Can you work these out from the model? Positions are in its coordinate system, mm. Round coordinates to 2 decimals unless told otherwise and drop trailing zeros. Loops run counter-clockwise (first coordinate to the right, second up) from the corner with the lowest first, then second, coordinate; pieces in that order, holes last. Notation, with made-up numbers: M 53,4.5 L 103,4.5 A19 ccw 103,31.5 Z; hole C -10,-33.5 d6. An arc over 180 degrees is marked long. Return JSON: item names as keys, results as strings.
```python
from build123d import *

# Parameters (mm, degrees)
BOSS_EXTRUDE1_DEPTH      = 1.5875
BOSS_EXTRUDE1_DEPTH_BACK = 1.5875
SKETCH1_W                = 6.35
SKETCH1_H                = 19.05
SKETCH1_R                = 1.5875
FILLET1_R                = 3.175


with BuildPart() as part:
    # Sketch1 → Boss-Extrude1 (new, two sides: drawn at the far end of the back side and taken through both)
    with BuildSketch(Plane(origin=(0, 0, 0), x_dir=(0, 0, -1), z_dir=(1, 0, 0)).offset(-BOSS_EXTRUDE1_DEPTH_BACK)):
        with Locations((0, -6.35)):
            Rectangle(SKETCH1_W, SKETCH1_H)
        Circle(SKETCH1_R, mode=Mode.SUBTRACT)
        with Locations((0, -12.7)):
            Circle(SKETCH1_R, mode=Mode.SUBTRACT)
    extrude(amount=BOSS_EXTRUDE1_DEPTH + BOSS_EXTRUDE1_DEPTH_BACK)

    # Fillet1
    fillet1_edges = [part.edges().sort_by_distance(p)[0] for p in [
        (0, -15.875, -3.175),
        (0, -15.875, 3.175),
        (0, 3.175, -3.175),
        (0, 3.175, 3.175),
    ]]
    fillet(fillet1_edges, radius=FILLET1_R - 0.0001)  # a hair under: the kernel refuses the full size


solid = part.part
```
Q1. Suppose I cut it at D-D, the plane z = 0.5. Please give me the cut outline in (x, y), plus the area to 3 significant figures.
Results:
{"outline": "M -1.59,-15.84 L 1.59,-15.84 L 1.59,-14.21 L -1.59,-14.21 Z; M -1.59,-11.19 L 1.59,-11.19 L 1.59,-1.51 L -1.59,-1.51 Z; M -1.59,1.51 L 1.59,1.51 L 1.59,3.14 L -1.59,3.14 Z", "area": "41.1 mm2"}
Q2. Suppose I cut it at B-B, the plane z = -1. Please give me the cut outline in (x, y).
Results:
{"outline": "M -1.59,-15.71 L 1.59,-15.71 L 1.59,-13.93 L -1.59,-13.93 Z; M -1.59,-11.47 L 1.59,-11.47 L 1.59,-1.23 L -1.59,-1.23 Z; M -1.59,1.23 L 1.59,1.23 L 1.59,3.01 L -1.59,3.01 Z"}
Q3. If I drill on line 1 along Y through (x, z) = (0.25, 0) (1 decimal); line 2 along Y through (x, z) = (0, 0.5); line 3 along Y through (x, z) = (-1.3, 2.75), over which ranges is the centre line in solid material (lowest first)?
Results:
{"line 1": "y = -15.9 to -14.3, -11.1 to -1.6, 1.6 to 3.2", "line 2": "y = -15.84 to -14.21, -11.19 to -1.51, 1.51 to 3.14", "line 3": "y = -14.29 to 1.59"}
Q4. Suppose I cut it at C-C, the plane y = -12.5. Please give me the cut outline in (x, z) (1 decimal), plus the area to 3 significant figures.
Results:
{"outline": "M -1.6,-3.2 L 1.6,-3.2 L 1.6,-1.6 L -1.6,-1.6 Z; M -1.6,1.6 L 1.6,1.6 L 1.6,3.2 L -1.6,3.2 Z", "area": "10.2 mm2"}
Q5. Suppose I cut it at A-A, the plane x = -1.3. State how many separate pieces and enclosed holes the cut face has, plus the area to 3 significant figures.
Results:
{"separate pieces": "1", "enclosed holes": "2", "area": "96.5 mm2"}
Q6. Thinking about a two-plate mould opening in Y: for faces 1 (the cylindrical face through (0.02, -14.92, 2.27)), 2 (the cylindrical face through (-0.022, -11.126, 0.207)), 3 (the cylindrical face through (0.02, 2.22, 2.27)), 4 (the flat face through (0, -6, 3.175)), which applies, pulls with the +Y half, pulls with the -Y half, needs draft (parallel to the pull), parting line crosses it, or undercut?
Results:
{"face 1": "pulls with the -Y half", "face 2": "undercut", "face 3": "pulls with the +Y half", "face 4": "needs draft"}
